Source: CAD feature listing. Evaluate the final solid. Frame: model axes, mm. Give positions to 0.01 mm unless a question says otherwise; leave off trailing zeros. Order: outer loops, then holes, each group sorted by start corner. A loop starts at its lowest first (then second) coordinate and runs counter-clockwise, first axis right, second up. Notation, with made-up numbers: (4, 65) -> (24, 65) arc R4 cw to (24, 72) -> close; hole circle Ø8 at (41, 5). An arc over 180 degrees is marked (long way). Use one line per item in the form item = value. Start each with the question number.
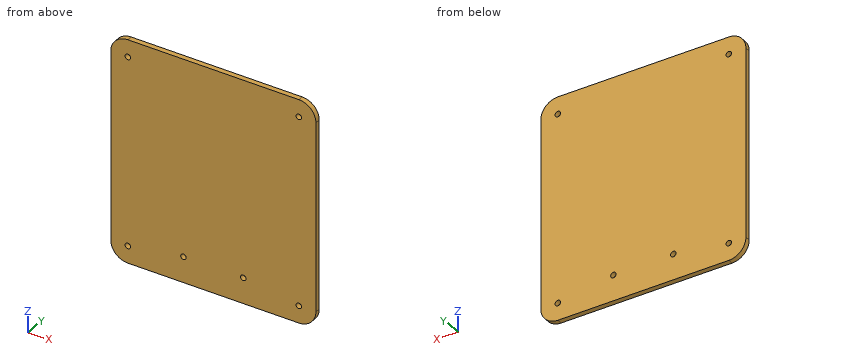
from build123d import *

# Parameters (mm, degrees)
SKETCH1_R           = 1.6
BOSS_EXTRUDE1_DEPTH = 3
SKETCH2_R           = 1.6
CUT_EXTRUDE1_DEPTH  = 89.509886453


with BuildPart() as part:
    # Sketch1 → Boss-Extrude1 (new body)
    with BuildSketch(Plane(origin=(0, 0, 0), x_dir=(1, 0, 0), z_dir=(0, 1, 0))):
        with BuildLine():
            Line((-50, 65), (50, 65))
            ThreePointArc((50, 65), (57.071067812, 62.071067812), (60, 55))
            Line((60, 55), (60, -55))
            ThreePointArc((60, -55), (57.071067812, -62.071067812), (50, -65))
            Line((50, -65), (-50, -65))
            ThreePointArc((-50, -65), (-57.071067812, -62.071067812), (-60, -55))
            Line((-60, -55), (-60, 55))
            ThreePointArc((-60, 55), (-57.071067812, 62.071067812), (-50, 65))
        make_face()
        with Locations(Location((50, -55, 0), (0, 0, 90))):
            Circle(SKETCH1_R, mode=Mode.SUBTRACT)
        with Locations(Location((-50, -55, 0), (0, 0, 270))):
            Circle(SKETCH1_R, mode=Mode.SUBTRACT)
        with Locations(Location((50, 55, 0), (0, 0, 270))):
            Circle(SKETCH1_R, mode=Mode.SUBTRACT)
        with Locations(Location((-50, 55, 0), (0, 0, 90))):
            Circle(SKETCH1_R, mode=Mode.SUBTRACT)
    extrude(amount=BOSS_EXTRUDE1_DEPTH)

    # Sketch2 → Cut-Extrude1 (cut, through all)
    with BuildSketch(Plane(origin=(0, 3, 0), x_dir=(1, 0, 0), z_dir=(0, 1, 0))):
        with Locations(Location((-17.5, 50, 0), (0, 0, 270))):
            Circle(SKETCH2_R)
        with Locations(Location((17.5, 50, 0), (0, 0, 270))):
            Circle(SKETCH2_R)
    extrude(amount=-CUT_EXTRUDE1_DEPTH, mode=Mode.SUBTRACT)


solid = part.part
1) Material intervals for probe 1 along X at (y, z) = (1.2, -50); probe 2 along X at (y, z) = (0.9, 55); probe 3 along Z at (x, y) = (-49, 0.35), sorted ascending.
2) Cut plane A-A, the plane z = -50. Return the cut outline in (x, y), plus the area to 3 significant figures.
3) Cut plane B-B, the plane x = -17.5. Return the cut outline in (y, z), plus the area to 3 significant figures.
Output values:
q1.probe_1 = -60 to -19.1, -15.9 to 15.9, 19.1 to 60
q1.probe_2 = -60 to -51.6, -48.4 to 48.4, 51.6 to 60
q1.probe_3 = -65 to -56.25, -53.75 to 53.75, 56.25 to 65
q2.outline = (-60, 0) -> (-19.1, 0) -> (-19.1, 3) -> (-60, 3) -> close; (-15.9, 0) -> (15.9, 0) -> (15.9, 3) -> (-15.9, 3) -> close; (19.1, 0) -> (60, 0) -> (60, 3) -> (19.1, 3) -> close
q2.area = 341 mm^2
q3.outline = (0, -65) -> (3, -65) -> (3, -51.6) -> (0, -51.6) -> close; (0, -48.4) -> (3, -48.4) -> (3, 65) -> (0, 65) -> close
q3.area = 380 mm^2
